Geometry: final body of the model. Coordinates: model frame, mm. A direction names the side the tool comes from. Coordinates: 2 decimals unless noted, no trailing zeros. Loops run counter-clockwise (first coordinate to the right, second up) from the corner with the lowest first, then second, coordinate; pieces in that order, holes last. Notation, with made-up numbers: (54, 11.25) - (105, 11.25) arc R8 ccw to (105, 25.25) - close; hole circle Ø6 at (84, 55). An arc over 180 degrees is marked (long way). Return JSON: item names as keys, results as strings.
from build123d import *

# Parameters (mm, degrees)
SKETCH1_W           = 182.5625
SKETCH1_H           = 111.125
BOSS_EXTRUDE1_DEPTH = 4.7625
BOSS_EXTRUDE2_DEPTH = 25.4


with BuildPart() as part:
    # Sketch1 → Boss-Extrude1 (new body)
    with BuildSketch(Plane(origin=(0, 0, 0), x_dir=(1, 0, 0), z_dir=(0, 1, 0))):
        with Locations((9.695676813, -15.715633096)):
            Rectangle(SKETCH1_W, SKETCH1_H)
    extrude(amount=BOSS_EXTRUDE1_DEPTH)

    # Sketch3 → Boss-Extrude2 (add)
    with BuildSketch(Plane.XZ):
        Polygon((-86.348073187, -39.846866904), (-86.348073187, -20.796866904), (-81.585573187, -20.796866904), (-81.585573187, -39.846866904), (100.976926813, -39.846866904), (100.976926813, -44.609366904), (-86.348073187, -44.609366904), align=None)
        Polygon((-86.348073187, 71.278133096), (-86.348073187, 52.228133096), (-81.585573187, 52.228133096), (-81.585573187, 71.278133096), (100.976926813, 71.278133096), (100.976926813, 76.040633096), (-81.585573187, 76.040633096), (-86.348073187, 76.040633096), align=None)
    extrude(amount=-BOSS_EXTRUDE2_DEPTH)


solid = part.part
Item 1: Section query C-C, the plane x = 39.5. Return loops of the section in (y, z).
Worked out:
{"outline": "(0, -44.61) - (25.4, -44.61) - (25.4, -39.85) - (4.76, -39.85) - (4.76, 71.28) - (25.4, 71.28) - (25.4, 76.04) - (0, 76.04) - close"}
Item 2: Section query A-A, the plane y = 21.25. Return loops of the section in (x, z).
Worked out:
{"outline": "(-86.35, -44.61) - (100.98, -44.61) - (100.98, -39.85) - (-81.59, -39.85) - (-81.59, -20.8) - (-86.35, -20.8) - close; (-86.35, 52.23) - (-81.59, 52.23) - (-81.59, 71.28) - (100.98, 71.28) - (100.98, 76.04) - (-86.35, 76.04) - close"}
Item 3: Mould query, pull axis Z, two halves, no side actions, for faces 4 (the face through (-84, 13, 52.228)), 5 (the face through (-86.348, 13, -33)), 6 (the face through (9, 13, 76.041)). Classes: +Z half, -Z half, draft (parallel to the pull), parting line (faces both ways), or undercut.
Worked out:
{"face 4": "undercut", "face 5": "draft", "face 6": "+Z half"}
Item 4: Section query D-D, the plane y = 2.5. Return loops of the section in (x, z), and give its area (3 significant figures).
Worked out:
{"outline": "(-86.35, -44.61) - (100.98, -44.61) - (100.98, 76.04) - (-86.35, 76.04) - (-86.35, 52.23) - (-81.59, 52.23) - (-81.59, -20.8) - (-86.35, -20.8) - close", "area": "22,300 mm^2"}
Item 5: First-contact query: pin 1 Ø12 at (x, z) = (-1.5, 20.5) entering from +Y; pin 2 Ø4 at (y, z) = (2.5, 30.5) entering from -X; pin 3 Ø5.5 at (y, z) = (15.5, 59) entering from +X. Flat tips, straight axial feed; report the tip coordinate or a pass-through.
Worked out:
{"pin 1": "y = 4.76", "pin 2": "x = -81.59", "pin 3": "x = -81.59"}
Item 6: Section query B-B, the plane z = -25.5. Return loops of the section in (x, y), and give its area (3 significant figures).
Worked out:
{"outline": "(-86.35, 0) - (100.98, 0) - (100.98, 4.76) - (-81.59, 4.76) - (-81.59, 25.4) - (-86.35, 25.4) - close", "area": "990 mm^2"}
Item 7: Ray query, probe 1 along Z at (x, y) = (-24, 21.5); probe 2 along Y at (x, z) = (-71.5, 60.5); probe 3 along X at (y, z) = (18.5, -26). Return the intervals inside material, ascending. Write a range as from..to.
Worked out:
{"probe 1": "-44.61..-39.85, 71.28..76.04", "probe 2": "0..4.76", "probe 3": "-86.35..-81.59"}
Item 8: Reachability of faces 1 (the face through (-86.348, 13, 64)), 2 (the face through (-84, 13, -20.797)), 3 (the face through (8, 15, 71.278)) from +Z, -Z, +X, -X, +Y, -Y: full face, straight path, thin tool, end or side. Return the list, or none.
Worked out:
{"face 1": "+Z, -Z, -X, +Y, -Y", "face 2": "-X, +Y, -Y", "face 3": "+X, +Y"}
